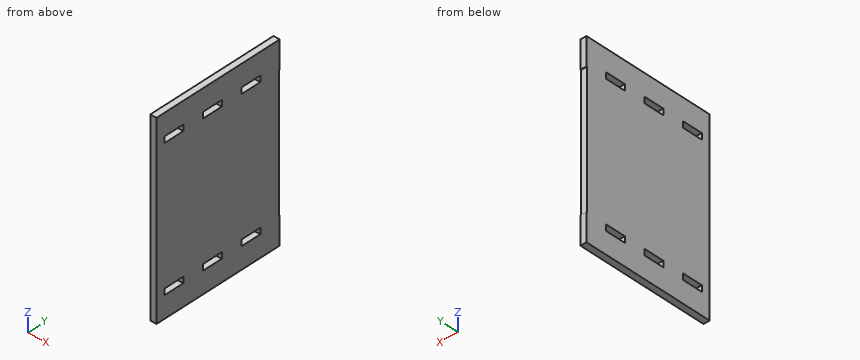
from build123d import *

# Parameters (mm, degrees)
SKETCH1_W           = 90
SKETCH1_H           = 64
BOSS_EXTRUDE1_DEPTH = 3
SKETCH2_W           = 2.9
SKETCH2_H           = 9.8
CUT_EXTRUDE1_DEPTH  = 3
SKETCH4_W           = 63.5
SKETCH4_H           = 0.25
CUT_EXTRUDE2_DEPTH  = 10


with BuildPart() as part:
    # Sketch1 → Boss-Extrude1 (new body)
    with BuildSketch(Plane(origin=(0, 0, 0), x_dir=(0, 0, -1), z_dir=(1, 0, 0))):
        Rectangle(SKETCH1_W, SKETCH1_H)
    extrude(amount=BOSS_EXTRUDE1_DEPTH)

    # Sketch2 → Cut-Extrude1 (cut)
    with BuildSketch(Plane(origin=(3, 0, 0), x_dir=(0, 0, -1), z_dir=(1, 0, 0))):
        with Locations((-33.2, 17)):
            Rectangle(SKETCH2_W, SKETCH2_H)
        with Locations((-33.2, -3)):
            Rectangle(SKETCH2_W, SKETCH2_H)
        with Locations((-33.2, -23)):
            Rectangle(SKETCH2_W, SKETCH2_H)
        with Locations((33.2, -23)):
            Rectangle(SKETCH2_W, SKETCH2_H)
        with Locations((33.2, -3)):
            Rectangle(SKETCH2_W, SKETCH2_H)
        with Locations((33.2, 17)):
            Rectangle(SKETCH2_W, SKETCH2_H)
    extrude(amount=-CUT_EXTRUDE1_DEPTH, mode=Mode.SUBTRACT)

    # Sketch4 → Cut-Extrude2 (cut)
    with BuildSketch(Plane(origin=(3, 0, 0), x_dir=(0, 0, -1), z_dir=(1, 0, 0))):
        with Locations((0, 31.875)):
            Rectangle(SKETCH4_W, SKETCH4_H)
    extrude(amount=-CUT_EXTRUDE2_DEPTH, mode=Mode.SUBTRACT)


solid = part.part
Build history of the part. All positions in model axes, mm. Round coordinates to 2 decimals unless told otherwise and drop trailing zeros. Loops run counter-clockwise (first coordinate to the right, second up) from the corner with the lowest first, then second, coordinate; pieces in that order, holes last. Notation, with made-up numbers: (25, 56) -> (81, 56) arc R19 ccw to (81, 66) -> close; hole circle Ø10 at (-37, -34.75). An arc over 180 degrees is marked (long way). Answer in a Markdown table with one row per item.
Item 1: Pin check, flat tips, straight feed: pin 1 (12 mm diameter, centred on y = 20.5, z = -21, fed in from -X); pin 2 (1 mm diameter, centred on x = 2, z = 0.5, fed in from +Y). Stop position of each tip, or through.
Answers below:
| item | result |
|---|---|
| pin 1 | stops at x = 0 |
| pin 2 | stops at y = 31.75 |
Item 2: Drill centre lines: L1, parallel to Y at x = 1.55, z = -33; L2, parallel to Z at x = 2.85, y = 0; L3, parallel to Y at x = 1.5, z = -27. Where is each one in solid material? Low to high. Write a range as [from, to].
Answers below:
| item | result |
|---|---|
| L1 | y = [-32, -27.9], [-18.1, -7.9], [1.9, 12.1], [21.9, 32] |
| L2 | z = [-45, -34.65], [-31.75, 31.75], [34.65, 45] |
| L3 | y = [-32, 31.75] |
Item 3: Saw through at A-A (y = -0.5). Write the cut outline in (x, z).
Answers below:
| item | result |
|---|---|
| outline | (0, -45) -> (3, -45) -> (3, -34.65) -> (0, -34.65) -> close; (0, -31.75) -> (3, -31.75) -> (3, 31.75) -> (0, 31.75) -> close; (0, 34.65) -> (3, 34.65) -> (3, 45) -> (0, 45) -> close |
Item 4: Saw through at B-B (x = 1.1). State how many separate pieces and enclosed holes the cut face has, and give its area (3 significant figures).
Answers below:
| item | result |
|---|---|
| separate pieces | 1 |
| enclosed holes | 6 |
| area | 5,570 mm² |
